from build123d import *

# Parameters (mm, degrees)
SKETCH1_R           = 1.3
SKETCH1_R_2         = 1.5
BOSS_EXTRUDE1_DEPTH = 3


with BuildPart() as part:
    # Sketch1 → Boss-Extrude1 (new body)
    with BuildSketch(Plane.XY):
        with BuildLine():
            Line((-67.43171984, 21.978952762), (-67.43171984, -48.021047238))
            Line((-67.43171984, -48.021047238), (42.56828016, -48.021047238))
            ThreePointArc((42.56828016, -48.021047238), (77.56828016, -13.021047238), (42.56828016, 21.978952762))
            Line((42.56828016, 21.978952762), (-67.43171984, 21.978952762))
        make_face()
        with Locations((-58.93171984, 14.978952762)):
            Circle(SKETCH1_R, mode=Mode.SUBTRACT)
        with Locations((34.06828016, 14.978952762)):
            Circle(SKETCH1_R_2, mode=Mode.SUBTRACT)
        with Locations((34.104880448, -41.021035277)):
            Circle(SKETCH1_R_2, mode=Mode.SUBTRACT)
        with Locations((-58.895119552, -41.021035277)):
            Circle(SKETCH1_R_2, mode=Mode.SUBTRACT)
    extrude(amount=BOSS_EXTRUDE1_DEPTH)


solid = part.part
Check sheet for the modelled part. Datum: model origin and axes. Units: mm. Round coordinates to 2 decimals unless told otherwise and drop trailing zeros. Loops run counter-clockwise (first coordinate to the right, second up) from the corner with the lowest first, then second, coordinate; pieces in that order, holes last. Notation, with made-up numbers: (57, -12.75) - (108, -12.75) arc R23 ccw to (108, 4.25) - close; hole circle Ø2 at (44, 22). An arc over 180 degrees is marked (long way). Answer as CSV lines item,"result". Start each with the question number.
Item 1: Section check B-B (x = 52). Record the boundary of the cut face in (y, z).
Item 2: Section check A-A (z = 2.5). Record the boundary of the cut face in (x, y).
Item 3: Section check C-C (y = -35.5). Record the boundary of the cut face in (x, z).
Item 4: Scan lines: line 1 (X direction, y = 16, z = 2.85); line 2 (X direction, y = -35.5, z = 1.1); line 3 (Y direction, x = 48.5, z = 0.75). Record each from-to range of solid material in increasing order. Write a range as [from, to].
Item 5: Depth check by flat-ended pin: P1, Ø6, axis at x = -31, y = -32.5, coming from the -Z side; P2, Ø1.8, axis at x = -58.9, y = -41.02, coming from the +Z side. Enter the tip coordinate at first touch or a pass-through.
Item 6: Release check for a two-part mould opening along X. For faces 1 (the cylindrical face through (-60.09, -41.93, 1.48)), 2 (the flat face through (4, -13, 0)), 3 (the cylindrical face through (77.56, -13.79, 1.48)), 4 (the cylindrical face through (35.49, -41.6, 1.48)) record: +X half, -X half, draft (parallel to the pull), parting line (faces both ways), or undercut.
Report:
1,outline,"(-46.73, 0) - (20.68, 0) - (20.68, 3) - (-46.73, 3) - close"
2,outline,"(-67.43, -48.02) - (42.57, -48.02) arc R35 ccw to (42.57, 21.98) - (-67.43, 21.98) - close; hole circle Ø3 at (-58.9, -41.02); hole circle Ø2.6 at (-58.93, 14.98); hole circle Ø3 at (34.07, 14.98); hole circle Ø3 at (34.1, -41.02)"
3,outline,"(-67.43, 0) - (69.4, 0) - (69.4, 3) - (-67.43, 3) - close"
4,line 1,"x = [-67.43, -59.74], [-58.13, 32.97], [35.17, 62.13]"
4,line 2,"x = [-67.43, 69.4]"
4,line 3,"y = [-47.51, 21.47]"
5,P1,"stops at z = 0"
5,P2,"passes through"
6,face 1,"undercut"
6,face 2,"draft"
6,face 3,"+X half"
6,face 4,"undercut"
